from build123d import *

# Parameters (mm, degrees)
SKETCH1_R               = 375
BOSS_EXTRUDE1_DEPTH     = 30
SKETCH1_7_R             = 410
BOSS_EXTRUDE2_DEPTH     = 35
CUT_EXTRUDE1_DEPTH      = 36
CUT_EXTRUDE1_DEPTH_BACK = 31
CUT_EXTRUDE2_START      = 35
SKETCH1_14_R            = 315
CUT_EXTRUDE2_DEPTH      = 30
FILLET1_R               = 15
FILLET2_R               = 10


with BuildPart() as part:
    # Sketch1 → Boss-Extrude1 (new body)
    with BuildSketch(Plane(origin=(0, 0, 0), x_dir=(1, 0, 0), z_dir=(0, 1, 0))):
        Circle(SKETCH1_R)
    extrude(amount=-BOSS_EXTRUDE1_DEPTH)

    # Sketch1<7> → Boss-Extrude2 (add)
    with BuildSketch(Plane(origin=(0, 0, 0), x_dir=(1, 0, 0), z_dir=(0, 1, 0))):
        Circle(SKETCH1_7_R)
    extrude(amount=BOSS_EXTRUDE2_DEPTH)

    # Sketch1<10> → Cut-Extrude1 (cut, two sides)
    with BuildSketch(Plane(origin=(0, 0, 0), x_dir=(1, 0, 0), z_dir=(0, 1, 0))) as cut_extrude1_sk:
        with BuildLine():
            Line((-80, 220), (-80, 60))
            ThreePointArc((-80, 60), (-120, 20), (-160, 60))
            Line((-160, 60), (-160, 220))
            ThreePointArc((-160, 220), (-120, 260), (-80, 220))
        make_face()
        with BuildLine():
            Line((-80, -220), (-80, -60))
            ThreePointArc((-80, -60), (-120, -20), (-160, -60))
            Line((-160, -60), (-160, -220))
            ThreePointArc((-160, -220), (-120, -260), (-80, -220))
        make_face()
        with BuildLine():
            Line((80, 220), (80, 60))
            ThreePointArc((80, 60), (120, 20), (160, 60))
            Line((160, 60), (160, 220))
            ThreePointArc((160, 220), (120, 260), (80, 220))
        make_face()
        with BuildLine():
            Line((80, -220), (80, -60))
            ThreePointArc((80, -60), (120, -20), (160, -60))
            Line((160, -60), (160, -220))
            ThreePointArc((160, -220), (120, -260), (80, -220))
        make_face()
    extrude(amount=CUT_EXTRUDE1_DEPTH, mode=Mode.SUBTRACT)
    extrude(cut_extrude1_sk.sketch, amount=-CUT_EXTRUDE1_DEPTH_BACK, mode=Mode.SUBTRACT)

    # Sketch1<14> → Cut-Extrude2 (cut)
    with BuildSketch(Plane(origin=(0, 0, 0), x_dir=(1, 0, 0), z_dir=(0, 1, 0)).offset(CUT_EXTRUDE2_START)):
        Circle(SKETCH1_14_R)
    extrude(amount=-CUT_EXTRUDE2_DEPTH, mode=Mode.SUBTRACT)

    # Fillet1
    fillet1_edges = [part.edges().sort_by_distance(p)[0] for p in [
        (-410, 35, 0),
    ]]
    fillet(fillet1_edges, radius=FILLET1_R)

    # Fillet2
    fillet2_edges = [part.edges().sort_by_distance(p)[0] for p in [
        (-315, 35, 0),
    ]]
    fillet(fillet2_edges, radius=FILLET2_R)


solid = part.part
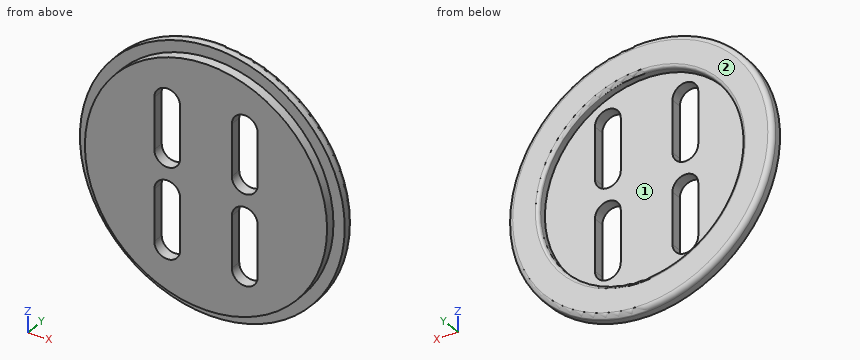
The listing builds one solid part. Answer for the finished solid, in the listing's coordinates (mm). Face numbers are marked on the shaded views. Round coordinates to 2 decimals unless told otherwise and drop trailing zeros. Write each loop counter-clockwise with the first axis right and the second up, starting at its lowest first coordinate (ties: lowest second). Pieces come first, ordered by that corner, then holes. Notation, with made-up numbers: M -33,27 L -26,27 A27 cw -26,64 Z; hole C 59,-22 d3. An arc over 180 degrees is marked long. Write each question's results on one line, items separated by ' | '. Start each with the question number.
Item 1: Find section A-A on y = -9.5. Write down the section's boundary in (x, z), and give its area (3 significant figures).
Item 2: Find section C-C on x = 120. Give the number of separate pieces and of enclosed holes in the cut face, and give its area (3 significant figures).
Item 3: Straight lines are drawn through the part: probe 1 along Z at (x, y) = (0, 19.75); probe 2 along X at (y, z) = (-20.5, 148.5). For each, find the intervals that lie inside material, in ascending order.
Item 4: The mould has two halves that part along Z. Classify the marked faces 1 and 2: +Z half, -Z half, draft (parallel to the pull), parting line (faces both ways), or undercut.
Item 5: Find section B-B on z = 0. Write down the section's boundary in (x, y).
Item 6: Given pin 1 Ø6 at (y, z) = (-5.5, 319) entering from +X; pin 2 Ø17.5 at (y, z) = (-15, 111) entering from +X; pin 3 Ø10.5 at (y, z) = (-17, -131.5) entering from +X, each flat-ended and moving along its own axis, determine where each tip first touches the part or whether it passes through.
Answer block:
1) outline: C 0,0 d750; hole M -160,-220 A40 ccw -80,-220 L -80,-60 A40 ccw -160,-60 Z; hole M -160,60 A40 ccw -80,60 L -80,220 A40 ccw -160,220 Z; hole M 80,-220 A40 ccw 160,-220 L 160,-60 A40 ccw 80,-60 Z; hole M 80,60 A40 ccw 160,60 L 160,220 A40 ccw 80,220 Z | area: 370,000 mm²
2) separate pieces: 3 | enclosed holes: 0 | area: 14,300 mm²
3) probe 1: z = -410 to -315, 315 to 410 | probe 2: x = -344.34 to -160, -80 to 80, 160 to 344.34
4) face 1: undercut | face 2: draft
5) outline: M -410,0 L -375,0 L -375,-30 L 375,-30 L 375,0 L 410,0 L 410,20 A15 ccw 395,35 L 325,35 A10 ccw 315,25 L 315,5 L -315,5 L -315,25 A10 ccw -325,35 L -395,35 A15 ccw -410,20 Z
6) pin 1: stops at x = 201.91 | pin 2: stops at x = 360.79 | pin 3: stops at x = 353.11
